Model file for the job. Use its own axes, mm. A direction names the side the tool comes from. Give positions to 0.01 mm unless a question says otherwise; leave off trailing zeros. Write each loop counter-clockwise with the first axis right and the second up, starting at its lowest first coordinate (ties: lowest second). Pieces come first, ordered by that corner, then holes. Notation, with made-up numbers: (-36, -38) - (0, -38) arc R29 ccw to (0, -10) - close; hole circle Ø4 at (35.5, -19.75). An arc over 180 degrees is marked (long way). One line per item, written item: value. Start each with the question number.
(1) 3-axis set-ups, long thin cutter, end or side, ignore diameter. For faces 1 (the face through (0, 7, 0)), 2 (the face through (0, 90, -10)), 3 (the face through (11, 49, -20)), 4 (the face through (0, 79, -16)), 5 (the face through (0.112, 82.899, -11.876)): which of +Z, -Z, +X, -X, +Y, -Y reach the whole face in a straight line?
(2) Drop flat-ended pins along their axis: P1, Ø2.5, axis at y = 11, z = 5, coming from the -X side; P2, Ø8, axis at x = -7, y = 18.5, coming from the -Z side; P3, Ø8, axis at y = 81, z = -8, coming from the +X side; P4, Ø1.5, axis at x = -13.5, z = -9.5, coming from the -Y side. Give the stop position or say it passes through.
(3) Mould opens along X. For faces 6 (the face through (-12, 94, 0)), 7 (the face through (-2, 11, 0)), 8 (the face through (0, 9, 0)), 9 (the face through (15.5, 53, 0)) say: pulls with the +X half, pulls with the -X half, needs draft (parallel to the pull), parting line crosses it, or undercut.
(4) Cut at B-B, the plane y = 44.5. List the corners of the cut face in (x, z), and give its area (3 significant figures).
(5) Probe L1, parallel to Y at x = -10.75, z = 0; L2, parallel to X at y = 81, z = 14.5; L3, parallel to Y at x = -12, z = 0. List the from-to ranges inside material, lowest first.
(6) Cut at C-C, the plane z = 0. List the corners of the cut face in (x, y), and give its area (3 significant figures).
from build123d import *

# Parameters (mm, degrees)
SKETCH1_R               = 30
BOSS_EXTRUDE1_DEPTH     = 14
SKETCH2_R               = 11.05
CUT_EXTRUDE1_DEPTH      = 7
SKETCH5_W               = 7.5
SKETCH5_H               = 40
BOSS_EXTRUDE2_DEPTH     = 80
FILLET1_R               = 10
CUT_EXTRUDE3_DEPTH      = 109.656569061
CUT_EXTRUDE3_DEPTH_BACK = 109.656569061
SKETCH7_R               = 11.05
CUT_EXTRUDE4_START      = -5
CUT_EXTRUDE4_DEPTH      = 5
BOSS_EXTRUDE4_DEPTH     = 16
FILLET2_R               = 10


with BuildPart() as part:
    # Sketch1 → Boss-Extrude1 (new body)
    with BuildSketch(Plane(origin=(0, 0, 0), x_dir=(1, 0, 0), z_dir=(0, 1, 0))):
        with Locations(Location((0, 0, 0), (0, 0, 90))):
            Circle(SKETCH1_R)
    extrude(amount=BOSS_EXTRUDE1_DEPTH)

    # Sketch2 → Cut-Extrude1 (cut)
    with BuildSketch(Plane.XZ):
        with Locations(Location((0, 0, 0), (0, 0, 270))):
            Circle(SKETCH2_R)
    extrude(amount=-CUT_EXTRUDE1_DEPTH, mode=Mode.SUBTRACT)

    # Sketch5 → Boss-Extrude2 (add)
    with BuildSketch(Plane(origin=(0, 14, 0), x_dir=(1, 0, 0), z_dir=(0, 1, 0))):
        with Locations((-11.75, 0)):
            Rectangle(SKETCH5_W, SKETCH5_H)
        with Locations((11.75, 0)):
            Rectangle(SKETCH5_W, SKETCH5_H)
    extrude(amount=BOSS_EXTRUDE2_DEPTH)

    # Fillet1
    fillet1_edges = [part.edges().sort_by_distance(p)[0] for p in [
        (-11.75, 94, 20),
        (-11.75, 94, -20),
        (11.75, 94, 20),
        (11.75, 94, -20),
    ]]
    fillet(fillet1_edges, radius=FILLET1_R)

    # Sketch7 → Cut-Extrude3 (cut, two sides: drawn at the far end of the back side and taken through both)
    with BuildSketch(Plane.ZY.offset(15.5).offset(-CUT_EXTRUDE3_DEPTH_BACK)):
        with Locations((0, 79)):
            Circle(SKETCH7_R)
    extrude(amount=CUT_EXTRUDE3_DEPTH + CUT_EXTRUDE3_DEPTH_BACK, mode=Mode.SUBTRACT)

    # Sketch8 → Cut-Extrude4 (cut)
    with BuildSketch(Plane(origin=(0, 14, 0), x_dir=(1, 0, 0), z_dir=(0, 1, 0)).offset(CUT_EXTRUDE4_START)):
        with BuildLine():
            Line((2, 29.933259094), (2, -29.933259094))
            ThreePointArc((2, -29.933259094), (0, -30), (-2, -29.933259094))
            Line((-2, -29.933259094), (-2, 29.933259094))
            ThreePointArc((-2, 29.933259094), (0, 30), (2, 29.933259094))
        make_face()
    extrude(amount=CUT_EXTRUDE4_DEPTH, mode=Mode.SUBTRACT)

    # Sketch9 → Boss-Extrude4 (add)
    with BuildSketch(Plane.ZY.offset(-8)):
        with BuildLine():
            Line((-10, 86.5), (-10, 94))
            Line((-10, 94), (-20, 94))
            Line((-20, 94), (-20, 79))
            Line((-20, 79), (-12.5, 79))
            ThreePointArc((-12.5, 79), (-11.858541226, 82.952847075), (-10, 86.5))
        make_face()
    extrude(amount=BOSS_EXTRUDE4_DEPTH)

    # Fillet2
    fillet2_edges = [part.edges().sort_by_distance(p)[0] for p in [
        (0, 94, -20),
    ]]
    fillet(fillet2_edges, radius=FILLET2_R - 0.0001)  # a hair under: the kernel refuses the full size


solid = part.part
Answers follow:
1. face 1: -Y
1. face 2: +Z, +Y
1. face 3: -Z, +X, -X, +Y
1. face 4: +Z, -Z
1. face 5: +Z
2. P1: stops at x = -29.76
2. P2: stops at z = -20
2. P3: stops at x = 15.5
2. P4: stops at y = 0
3. face 6: needs draft
3. face 7: undercut
3. face 8: undercut
3. face 9: pulls with the +X half
4. outline: (-15.5, -20) - (-8, -20) - (-8, 20) - (-15.5, 20) - close; (8, -20) - (15.5, -20) - (15.5, 20) - (8, 20) - close
4. area: 600 mm²
5. L1: y = 7 to 67.95, 90.05 to 94
5. L2: x = -15.5 to -8, 8 to 15.5
5. L3: y = 0 to 67.95, 90.05 to 94
6. outline: (-30, 0) - (-11.05, 0) - (-11.05, 7) - (11.05, 7) - (11.05, 0) - (30, 0) - (30, 14) - (15.5, 14) - (15.5, 67.95) - (8, 67.95) - (8, 14) - (2, 14) - (2, 9) - (-2, 9) - (-2, 14) - (-8, 14) - (-8, 67.95) - (-15.5, 67.95) - (-15.5, 14) - (-30, 14) - close; (-15.5, 90.05) - (-8, 90.05) - (-8, 94) - (-15.5, 94) - close; (8, 90.05) - (15.5, 90.05) - (15.5, 94) - (8, 94) - close
6. area: 1,530 mm²
